Here's how the part is built. I have some questions about the finished solid (model axes, mm). A direction names the side the tool comes from. Round coordinates to 2 decimals unless told otherwise and drop trailing zeros. Write each loop counter-clockwise with the first axis right and the second up, starting at its lowest first coordinate (ties: lowest second). Pieces come first, ordered by that corner, then holes. Notation, with made-up numbers: (56.5, -28.75) -> (106.5, -28.75) arc R7 ccw to (106.5, -17.75) -> close; hole circle Ø8 at (-19.75, 37.5). An arc over 180 degrees is marked (long way). Answer in a Markdown table with one row per item.
from build123d import *

# Parameters (mm, degrees)
F0_R     = 16.15
F0_R_2   = 5.1
F0_R_3   = 5.15
F1_DEPTH = 15
F0_R_4   = 4.35
F2_DEPTH = 5
F3_R     = 10
F4_SIZE  = 1.5


with BuildPart() as f1:
    # F0 (on Front) → F1 (new body)
    with BuildSketch(Plane.XZ):
        with BuildLine():
            ThreePointArc((17.4720673077, -4.726189162), (35.3828933588, -2.6502475765), (21.2048683234, 8.4893587629))
            ThreePointArc((21.2048683234, 8.4893587629), (21.2879399951, 20.805683816), (10.6130350411, 14.6619741923))
            ThreePointArc((10.6130350411, 14.6619741923), (-17.0636591342, -6.0366826114), (17.4720673077, -4.726189162))
        make_face()
        Circle(F0_R, mode=Mode.SUBTRACT)
        with Locations((26, 0)):
            Circle(F0_R_2, mode=Mode.SUBTRACT)
        with Locations((17.7130288462, 14.6713533491)):
            Circle(F0_R_3, mode=Mode.SUBTRACT)
    extrude(amount=-F1_DEPTH)

    # F0 (on Front) → F2 (join)
    with BuildSketch(Plane.XZ):
        with BuildLine():
            ThreePointArc((17.4720673077, -4.726189162), (35.3828933588, -2.6502475765), (21.2048683234, 8.4893587629))
            ThreePointArc((21.2048683234, 8.4893587629), (21.2879399951, 20.805683816), (10.6130350411, 14.6619741923))
            ThreePointArc((10.6130350411, 14.6619741923), (-17.0636591342, -6.0366826114), (17.4720673077, -4.726189162))
        make_face()
        Circle(F0_R, mode=Mode.SUBTRACT)
        with Locations((26, 0)):
            Circle(F0_R_2, mode=Mode.SUBTRACT)
        with Locations((17.7130288462, 14.6713533491)):
            Circle(F0_R_3, mode=Mode.SUBTRACT)
        with Locations((26, 0)):
            Circle(F0_R_2)
        with Locations((26, 0)):
            Circle(F0_R_4, mode=Mode.SUBTRACT)
    extrude(amount=F2_DEPTH)

    # F3
    f3_edges = [f1.edges().sort_by_distance(p)[0] for p in [
        (10.613035, 5, 14.661974),
        (21.204868, 5, 8.489359),
        (17.472067, 5, -4.726189),
    ]]
    fillet(f3_edges, radius=F3_R)

    # F4
    f4_edges = [f1.edges().sort_by_distance(p)[0] for p in [
        (-17.286785, -5, -5.364427),
    ]]
    chamfer(f4_edges, length=F4_SIZE)


solid = f1.part
1) I need wall thicknesses on line 1 (X direction, y = 12.5, z = 3.5); line 2 (Z direction, x = 22, y = 8.5); line 3 (X direction, y = 3.75, z = 11). Which ranges of each line are inside material? Lowest first, please. Write a range as [from, to].
Response:
| item | result |
|---|---|
| line 1 | x = [-17.76, -15.77], [15.77, 22.29], [29.71, 35.1] |
| line 2 | z = [-9.11, -3.16], [3.16, 11.82], [17.53, 20.33] |
| line 3 | x = [-14.37, -11.82], [11.82, 14.1], [21.32, 27.21] |
2) We'd pull the mould along Z, two halves only. Please class faces 1 (the face through (20.09, 5.88, 21.36)), 2 (the face through (-3.501, 5.14, -15.766)), 3 (the face through (33.9, -4.74, -3.16)): +Z half, -Z half, draft (parallel to the pull), parting line (faces both ways), or undercut.
Response:
| item | result |
|---|---|
| face 1 | +Z half |
| face 2 | undercut |
| face 3 | parting line |
3) I want a section at A-A, the plane x = 0. List the corners of the cut face in (y, z) for me.
Response:
| item | result |
|---|---|
| outline | (-5, -16.6) -> (-3.5, -18.1) -> (15, -18.1) -> (15, -16.15) -> (-5, -16.15) -> close; (-5, 16.15) -> (15, 16.15) -> (15, 18.1) -> (-3.5, 18.1) -> (-5, 16.6) -> close |
4) I want a section at C-C, the plane y = 9.5. Count the separate pieces of the cut face and the enclosed holes in it, and give its area (3 significant figures).
Response:
| item | result |
|---|---|
| separate pieces | 1 |
| enclosed holes | 3 |
| area | 518 mm^2 |
5) I want a section at B-B, the plane z = 0. List the corners of the cut face in (x, y) for me.
Response:
| item | result |
|---|---|
| outline | (-18.1, -3.5) -> (-16.6, -5) -> (-16.15, -5) -> (-16.15, 15) -> (-18.1, 15) -> close; (16.15, -5) -> (21.65, -5) -> (21.65, 0) -> (20.9, 0) -> (20.9, 15) -> (16.15, 15) -> close; (30.35, -5) -> (34.25, -5) -> (35.75, -3.5) -> (35.75, 15) -> (31.1, 15) -> (31.1, 0) -> (30.35, 0) -> close |
6) For pin 1 (5 mm diameter, centred on x = 25, y = -1, fed in from -Z); pin 2 (2 mm diameter, centred on x = -9.5, y = 9.5, fed in from -Z); pin 3 (6 mm diameter, centred on x = -12, y = -1.5, fed in from -Z), each with a flat end and sliding along its axis, tell me the tip position at first contact or that it passes through.
Response:
| item | result |
|---|---|
| pin 1 | stops at z = -9.75 |
| pin 2 | stops at z = -15.98 |
| pin 3 | stops at z = -15.7 |
7) Which directions (+Z, -Z, +X, -X, +Y, -Y) give clear straight access to the entire face, cutting with the end or side of a thin tool? Please do faces 4 (the face through (-17.44, 5.88, -4.85)), 5 (the face through (20.905, 7.395, 0.224)).
Response:
| item | result |
|---|---|
| face 4 | +Y, -Y |
| face 5 | +Y |
